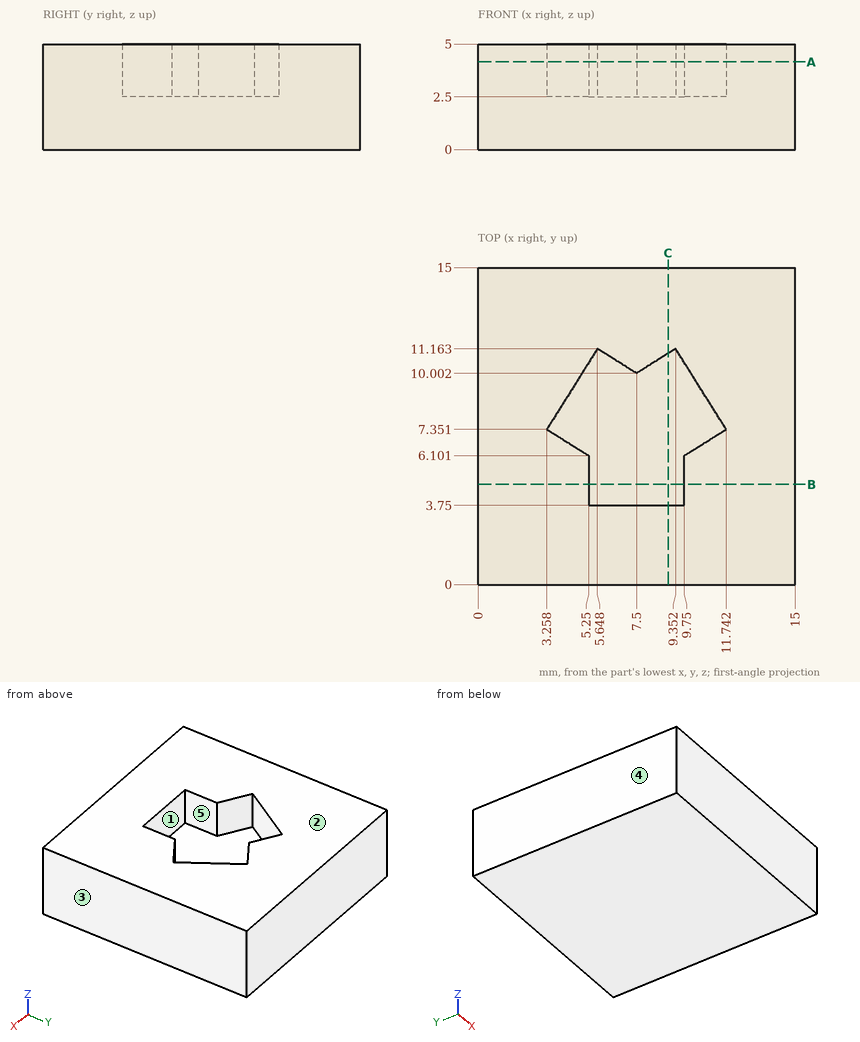
Drawing for the job (mm, zero at the part's lowest x, y, z). A direction names the side the tool comes from. Give positions to 0.01 mm unless a question says otherwise; leave off trailing zeros. Order: outer loops, then holes, each group sorted by start corner. A loop starts at its lowest first (then second) coordinate and runs counter-clockwise, first axis right, second up. Notation, with made-up numbers: M 51.5,63 L 103.5,63 A23 ccw 103.5,84 Z; hole C 85,-14 d2. An arc over 180 degrees is marked long. Put each result on its own line as item: value.
Item 1: Two-plate mould, pull along X, no slides. Class the marked faces 3, 4 and 5: +X half, -X half, draft (parallel to the pull), parting line (faces both ways), or undercut.
From the geometry:
face 3: +X half
face 4: -X half
face 5: undercut
Item 2: 3-axis set-ups, long thin cutter, end or side, ignore diameter. For the marked faces 1 and 2: which of +Z, -Z, +X, -X, +Y, -Y reach the whole face in a straight line?
From the geometry:
face 1: +Z
face 2: +Z, +X, -X, +Y, -Y
Item 3: Slice it at B-B, the plane y = 4.75. Write the cut outline in (x, z).
From the geometry:
outline: M 0,0 L 15,0 L 15,5 L 9.75,5 L 9.75,2.5 L 5.25,2.5 L 5.25,5 L 0,5 Z
Item 4: Slice it at A-A, the plane z = 4.15. Write the cut outline in (x, y).
From the geometry:
outline: M 0,0 L 15,0 L 15,15 L 0,15 Z; hole M 3.26,7.35 L 5.25,6.1 L 5.25,3.75 L 9.75,3.75 L 9.75,6.1 L 11.74,7.35 L 9.35,11.16 L 7.5,10 L 5.65,11.16 Z
Item 5: Slice it at C-C, the plane x = 9. Write the cut outline in (y, z).
From the geometry:
outline: M 0,0 L 15,0 L 15,5 L 10.94,5 L 10.94,2.5 L 3.75,2.5 L 3.75,5 L 0,5 Z
Item 6: Probe line 1 (X direction, y = 6, z = 3.5); line 2 (Z direction, x = 7.5, y = 5.75); line 3 (Y direction, x = 3.75, z = 4.1) (1 decimal). List the from-to ranges inside material, lowest first. Write a range as [from, to].
From the geometry:
line 1: x = [0, 5.25], [9.75, 15]
line 2: z = [0, 2.5]
line 3: y = [0, 7], [8.1, 15]
